Source: CAD feature listing. Evaluate the final solid. Frame: model axes, mm. Coordinates: 2 decimals unless noted, no trailing zeros. Write each loop counter-clockwise with the first axis right and the second up, starting at its lowest first coordinate (ties: lowest second). Pieces come first, ordered by that corner, then holes. Notation, with made-up numbers: M 18,48 L 47,48 A18 ccw 47,54 Z; hole C -15.75,64.25 d2. An arc over 180 degrees is marked long. Answer as CSV lines item,"result". Start each with the question number.
1. Line query: probe 1 along X at (y, z) = (0.8, 0); probe 2 along X at (y, z) = (2.1, -34); probe 3 along Z at (x, y) = (1.25, 3.05). Output: solid intervals per line, ascending. Write a range as [from, to].
2. Mould query, pull axis Z, two halves, no side actions, for faces 1 (the face through (-3, 4, -35)), 2 (the face through (4.25, 1.97, -33.53)). Classes: pulls with the +Z half, pulls with the -Z half, needs draft (parallel to the pull), parting line crosses it, or undercut.
3. Section C-C on z = -34. Return the cut outline in (x, y), plus the area to 3 significant figures.
4. Contact query for flat-ended pins moving along their axis: pin 1 Ø2.5 at (x, z) = (0, -68) entering from +Y; pin 2 Ø1 at (y, z) = (3, -24.5) entering from +X; pin 3 Ø2 at (x, y) = (-3, 3.5) entering from +Z. Output: stop coordinate, or through.
5. Section B-B on y = 1.85. Return the cut outline in (x, z) (3 decimals), plus the area to 3 significant figures.
6. Section A-A on x = 0. Return the cut outline in (y, z), plus the area to 3 significant figures.
7. Section D-D on z = -59. Return the cut outline in (x, y).
```python
from build123d import *

# Parameters (mm, degrees)
SKETCH1_R           = 1.5
BOSS_EXTRUDE1_DEPTH = 4


with BuildPart() as part:
    # Sketch1 → Boss-Extrude1 (new body)
    with BuildSketch(Plane(origin=(0, 0, 0), x_dir=(1, 0, 0), z_dir=(0, 1, 0))):
        with BuildLine():
            ThreePointArc((-5.48515199, 0.403865882), (0, -5.5), (5.48515199, 0.403865882))
            ThreePointArc((5.48515199, 0.403865882), (4.25, 34), (5.48515199, 67.596134118))
            ThreePointArc((5.48515199, 67.596134118), (0, 73.5), (-5.48515199, 67.596134118))
            ThreePointArc((-5.48515199, 67.596134118), (-4.25, 34), (-5.48515199, 0.403865882))
        make_face()
        Circle(SKETCH1_R, mode=Mode.SUBTRACT)
        with Locations((0, 68)):
            Circle(SKETCH1_R, mode=Mode.SUBTRACT)
        with Locations((0, 34)):
            Circle(SKETCH1_R, mode=Mode.SUBTRACT)
    extrude(amount=BOSS_EXTRUDE1_DEPTH)


solid = part.part
```
Values:
1,probe 1,"[-5.5, -1.5], [1.5, 5.5]"
1,probe 2,"[-4.25, -1.5], [1.5, 4.25]"
1,probe 3,"[-73.36, -68.83], [-67.17, -34.83], [-33.17, -0.83], [0.83, 5.36]"
2,face 1,"needs draft"
2,face 2,"undercut"
3,outline,"M -4.25,0 L -1.5,0 L -1.5,4 L -4.25,4 Z; M 1.5,0 L 4.25,0 L 4.25,4 L 1.5,4 Z"
3,area,"22.0 mm²"
4,pin 1,"through"
4,pin 2,"x = 4.36"
4,pin 3,"z = 5.12"
5,outline,"M -5.485,-67.596 A5.5 ccw long 5.485,-67.596 A457.525 cw 5.485,-0.404 A5.5 ccw long -5.485,-0.404 A457.525 cw Z; hole C 0,-68 d3; hole C 0,-34 d3; hole C 0,0 d3"
5,area,"709 mm²"
6,outline,"M 0,-73.5 L 4,-73.5 L 4,-69.5 L 0,-69.5 Z; M 0,-66.5 L 4,-66.5 L 4,-35.5 L 0,-35.5 Z; M 0,-32.5 L 4,-32.5 L 4,-1.5 L 0,-1.5 Z; M 0,1.5 L 4,1.5 L 4,5.5 L 0,5.5 Z"
6,area,"280 mm²"
7,outline,"M -4.93,0 L 4.93,0 L 4.93,4 L -4.93,4 Z"
